Verification items for the finished model (mm, model axes). A direction names the side the tool comes from. Give positions to 0.01 mm unless a question says otherwise; leave off trailing zeros. Order: outer loops, then holes, each group sorted by start corner. A loop starts at its lowest first (then second) coordinate and runs counter-clockwise, first axis right, second up. Notation, with made-up numbers: (52.5, -33.5) - (57.5, -33.5) arc R21 cw to (57.5, -16.5) - close; hole circle Ø4 at (-37.75, 52.5). An arc over 180 degrees is marked (long way). Answer as a JSON object with one key per item and string values.
```python
from build123d import *

# Parameters (mm, degrees)
F1_DEPTH = 6
F2_R     = 1
F4_DEPTH = 2.5
F6_DEPTH = 21
F7_R     = 1
F8_R     = 1


with BuildPart() as f1:
    # F0 (on Front) → F1 (new body)
    with BuildSketch(Plane.XZ):
        Polygon((0, 0), (0, -12.2), (-1.5, -12.2), (2.5, -17.1), (2.5, 0), (2.5, 2.5), (0, 2.5), (-16.5, 2.5), (-28.23, 2.5), (-39.96, 2.5), (-56.46, 2.5), (-58.96, 2.5), (-58.96, 0), (-58.96, -17.1), (-54.96, -12.2), (-56.46, -12.2), (-56.46, 0), (-46.36, 0), (-28.23, 0), (-10.1, 0), align=None)
    extrude(amount=F1_DEPTH)

    # F2
    f2_edges = [f1.edges().sort_by_distance(p)[0] for p in [
        (-58.96, -3, -17.1),
        (2.5, -3, -17.1),
        (-58.96, -3, 2.5),
        (2.5, -3, 2.5),
    ]]
    fillet(f2_edges, radius=F2_R)

    # F3 (on face) → F4 (join)
    with BuildSketch(Plane.XY.offset(2.5)):
        Polygon((-17.73, -6), (-38.73, -6), (-38.73, -29), (-28.23, -29), (-17.73, -29), align=None)
    extrude(amount=-F4_DEPTH)

    # F5 (on face) → F6 (join)
    with BuildSketch(Plane(origin=(-38.73, 0, 0), x_dir=(0, -1, 0), z_dir=(-1, 0, 0))):
        Polygon((31.5, 2.5), (29, 2.5), (29, -12.2), (27, -12.2), (31.5, -17.1), align=None)
    extrude(amount=-F6_DEPTH)

    # F7
    f7_edges = [f1.edges().sort_by_distance(p)[0] for p in [
        (-28.23, -31.5, -17.1),
    ]]
    fillet(f7_edges, radius=F7_R)

    # F8
    f8_edges = [f1.edges().sort_by_distance(p)[0] for p in [
        (-28.23, -31.5, 2.5),
    ]]
    fillet(f8_edges, radius=F8_R)


solid = f1.part
```
(1) Section check D-D (y = -20). Record the cut outline in (x, z).
Computed values:
{"outline": "(-38.73, 0) - (-17.73, 0) - (-17.73, 2.5) - (-38.73, 2.5) - close"}
(2) Gauge pin test, flat ends, axial feed: pin 1 Ø3.5 at (x, z) = (-30.5, -6.5) entering from +Y; pin 2 Ø14.5 at (x, y) = (-24.5, -11.5) entering from -Z. Record the tip position at first contact, or that the pin passes through.
Computed values:
{"pin 1": "stops at y = -29", "pin 2": "stops at z = 0"}
(3) Access from +Z, -Z, +X, -X, +Y, -Y to the whole of each face (thin tool, end or side, straight path). Record for faces 4 (the flat face through (-56.088, -2.958, -13.582)), 5 (the flat face through (0, -3, -6)), 6 (the flat face through (-52.6, -6, 0.2)).
Computed values:
{"face 4": "-Z, +Y, -Y", "face 5": "+Y, -Y", "face 6": "+Z, -Z, -X, -Y"}
(4) Section check A-A (z = -7). Record the cut outline in (x, y).
Computed values:
{"outline": "(-58.96, -6) - (-56.46, -6) - (-56.46, 0) - (-58.96, 0) - close; (-38.73, -31.5) - (-17.73, -31.5) - (-17.73, -29) - (-38.73, -29) - close; (0, -6) - (2.5, -6) - (2.5, 0) - (0, 0) - close"}
(5) Release check for a two-part mould opening along X. For faces 1 (the flat face through (-38.73, -23, 1)), 2 (the flat face through (-3.9, -6, 0.2)), 3 (the cylindrical face through (1.82, -3.04, -15.24)) record: pulls with the +X half, pulls with the -X half, needs draft (parallel to the pull), parting line crosses it, or undercut.
Computed values:
{"face 1": "pulls with the -X half", "face 2": "needs draft", "face 3": "undercut"}
(6) Material ranges on line 1 along X through (y, z) = (-2, -5.25); line 2 along X through (y, z) = (-5, -13.5); line 3 along Z through (x, y) = (-27.5, -18.5), recorded low to high. Write a range as [from, to].
Computed values:
{"line 1": "x = [-58.96, -56.46], [0, 2.5]", "line 2": "x = [-58.96, -56.02], [-0.44, 2.5]", "line 3": "z = [0, 2.5]"}
(7) Section check B-B (x = -24.5). Record the cut outline in (y, z), then the cut area to 3 significant figures.
Computed values:
{"outline": "(-31.5, -14.53) arc R1 ccw to (-29.76, -15.21) - (-27, -12.2) - (-29, -12.2) - (-29, 0) - (0, 0) - (0, 2.5) - (-30.5, 2.5) arc R1 ccw to (-31.5, 1.5) - close", "area": "119 mm²"}
(8) Section check C-C (z = -13.25). Record the cut outline in (x, y), then the cut area to 3 significant figures.
Computed values:
{"outline": "(-58.96, -6) - (-55.82, -6) - (-55.82, 0) - (-58.96, 0) - close; (-38.73, -31.5) - (-17.73, -31.5) - (-17.73, -27.96) - (-38.73, -27.96) - close; (-0.64, -6) - (2.5, -6) - (2.5, 0) - (-0.64, 0) - close", "area": "112 mm²"}
